Here's how the part is built. I have some questions about the finished solid (model axes, mm). Face numbers are marked on the shaded views. A direction names the side the tool comes from. Coordinates: 2 decimals unless noted, no trailing zeros. Order: outer loops, then holes, each group sorted by start corner. A loop starts at its lowest first (then second) coordinate and runs counter-clockwise, first axis right, second up. Notation, with made-up numbers: (-3, 84) - (25, 84) arc R22 cw to (25, 113) - close; hole circle Ø1 at (3, 61.25). An arc over 180 degrees is marked (long way). Answer in a Markdown table with one row per item. Add a question column.
Item 1: Will these pins go through, and if not, where does the flat tip stop? pin 1 Ø1 at (x, z) = (31.5, -20) entering from +Y; pin 2 Ø2 at (x, z) = (35, 1) entering from +Y; pin 3 Ø1.6 at (x, z) = (14.5, -32.5) entering from +Y.
Item 2: I want a section at A-A (z = 0). Please give me the cut outline in (x, y).
Item 3: I want a section at D-D (z = -30). Please give me the cut outline in (x, y), plus the area to 3 significant figures.
Item 4: I want a section at B-B (y = 5.5). Please give me the cut outline in (x, z) (3 decimals), plus the area to 3 significant figures.
Item 5: If I drill on line 1 along X through (y, z) = (0.7, 0); line 2 along X through (y, z) = (10.16, 10.5); line 3 along Z through (x, y) = (4.5, 15.5), over which ranges is the centre line in solid material (lowest first)? Write a range as from..to.
Item 6: I want a section at C-C (x = 38). Please give me the cut outline in (y, z) (3 decimals), plus the area to 3 significant figures.
Item 7: Thinking about a two-plate mould opening in X: for the marked faces 1, 2 and 3, which applies, +X half, -X half, draft (parallel to the pull), parting line (faces both ways), or undercut?
Item 8: On a 3-axis mill with a long thin cutter (end or side, diameter ignored), from which of +Z, -Z, +X, -X, +Y, -Y can I reach the whole of each face in a straight line? I mean the marked faces 4 and 5. Say none if no direction works.
```python
from build123d import *

# Parameters (mm, degrees)
SKETCH1_W               = 40.64
SKETCH1_H               = 17.526
BOSS_EXTRUDE1_DEPTH     = 37.211
CUT_EXTRUDE1_DEPTH      = 32.385
FILLET1_R               = 3.81
SKETCH3_W               = 3.175
SKETCH3_H               = 6.35
SKETCH3_W_2             = 19.05
CUT_EXTRUDE2_DEPTH      = 58.822390101
CHAMFER1_SIZE           = 10
CUT_EXTRUDE7_DEPTH      = 58.822390101
CUT_EXTRUDE7_DEPTH_BACK = 58.822390101
SKETCH5_R               = 1.5875
BOSS_EXTRUDE2_REACH     = 83.728
SKETCH6_W               = 2.032
SKETCH6_H               = 6.35
BOSS_EXTRUDE3_REACH     = 83.728
SKETCH7_W               = 2.032
SKETCH7_H               = 6.35


with BuildPart() as part:
    # Sketch1 → Boss-Extrude1 (new, symmetric)
    with BuildSketch(Plane.XY):
        with Locations((20.32, 8.763)):
            Rectangle(SKETCH1_W, SKETCH1_H)
    extrude(amount=BOSS_EXTRUDE1_DEPTH, both=True)

    # Sketch2 → Cut-Extrude1 (cut, symmetric)
    with BuildSketch(Plane.XY):
        with BuildLine():
            Line((19.304, 10.16), (19.304, 17.526))
            Line((19.304, 17.526), (15.578005168, 17.526))
            ThreePointArc((15.578005168, 17.526), (2.000497097, 6.032622095), (19.304, 10.16))
        make_face()
        with BuildLine():
            Line((21.336, 10.16), (21.336, 17.526))
            Line((21.336, 17.526), (25.061994832, 17.526))
            ThreePointArc((25.061994832, 17.526), (38.639502903, 6.032622095), (21.336, 10.16))
        make_face()
    extrude(amount=CUT_EXTRUDE1_DEPTH, both=True, mode=Mode.SUBTRACT)

    # Fillet1
    fillet1_edges = [part.edges().sort_by_distance(p)[0] for p in [
        (0, 17.526, 0),
        (40.64, 17.526, 0),
    ]]
    fillet(fillet1_edges, radius=FILLET1_R)

    # Sketch3 → Cut-Extrude2 (cut, through all)
    with BuildSketch(Plane(origin=(40.64, 0, 0), x_dir=(0, 0, -1), z_dir=(1, 0, 0))):
        with Locations((-33.0835, 14.351)):
            Rectangle(SKETCH3_W, SKETCH3_H)
        with Locations((0, 14.351)):
            Rectangle(SKETCH3_W_2, SKETCH3_H)
        with Locations((33.0835, 14.351)):
            Rectangle(SKETCH3_W, SKETCH3_H)
    extrude(amount=-CUT_EXTRUDE2_DEPTH, mode=Mode.SUBTRACT)

    # Chamfer1
    # the kernel refuses this chamfer: 10 mm, written as the material it takes off along each edge
    with BuildSketch(Plane(origin=(21.336, 17.526, -9.525), x_dir=(0, -0.9996219169112968, 0.027495876610586664), z_dir=(-1, 0, 0))) as chamfer1_piece_1_section:
        Polygon((CHAMFER1_SIZE * 0.999621916911, -CHAMFER1_SIZE * 0.0274958766106), (-CHAMFER1_SIZE * 0.0274958766106, -CHAMFER1_SIZE * 0.999621916911), (0, 0), align=None)
    chamfer1_piece_1 = extrude(amount=2.032, mode=Mode.PRIVATE)
    chamfer1_piece_1 = split(chamfer1_piece_1, bisect_by=Plane(origin=(20.32, 11.176, -13.183669109), z_dir=(0, 1, 0)), keep=Keep.TOP, mode=Mode.PRIVATE)
    add(chamfer1_piece_1, mode=Mode.SUBTRACT)
    with BuildSketch(Plane(origin=(21.336, 17.526, 9.525), x_dir=(0, 0.027495876610586324, 0.9996219169112968), z_dir=(-1, 0, 0))) as chamfer1_piece_2_section:
        Polygon((CHAMFER1_SIZE * 0.999621916911, -CHAMFER1_SIZE * 0.0274958766106), (-CHAMFER1_SIZE * 0.0274958766106, -CHAMFER1_SIZE * 0.999621916911), (0, 0), align=None)
    chamfer1_piece_2 = extrude(amount=2.032, mode=Mode.PRIVATE)
    chamfer1_piece_2 = split(chamfer1_piece_2, bisect_by=Plane(origin=(20.32, 11.176, 13.183669109), z_dir=(0, 1, 0)), keep=Keep.TOP, mode=Mode.PRIVATE)
    add(chamfer1_piece_2, mode=Mode.SUBTRACT)

    # Sketch5 → Cut-Extrude7 (cut, two sides: drawn at the far end of the back side and taken through both)
    with BuildSketch(Plane.XZ.offset(-CUT_EXTRUDE7_DEPTH_BACK)):
        with Locations(Location((30.423380261, 0, 0), (0, 0, 270))):
            Circle(SKETCH5_R)
        with Locations(Location((10.216619739, 0, 0), (0, 0, 270))):
            Circle(SKETCH5_R)
    extrude(amount=CUT_EXTRUDE7_DEPTH + CUT_EXTRUDE7_DEPTH_BACK, mode=Mode.SUBTRACT)

    # Sketch6 → Boss-Extrude2 (add, up to next)
    with BuildSketch(Plane(origin=(0, 0, -31.496), x_dir=(-1, 0, 0), z_dir=(0, 0, -1)), mode=Mode.PRIVATE) as boss_extrude2_sk1:
        with Locations((-20.32, 14.351)):
            Rectangle(SKETCH6_W, SKETCH6_H)
    boss_extrude2_tool1 = extrude(boss_extrude2_sk1.sketch, amount=BOSS_EXTRUDE2_REACH, mode=Mode.PRIVATE) - part.part
    add(boss_extrude2_tool1.solids().sort_by_distance((20.32, 14.351, -31.496))[0])

    # Sketch7 → Boss-Extrude3 (add, up to next)
    with BuildSketch(Plane.XY.offset(31.496), mode=Mode.PRIVATE) as boss_extrude3_sk1:
        with Locations((20.32, 14.351)):
            Rectangle(SKETCH7_W, SKETCH7_H)
    boss_extrude3_tool1 = extrude(boss_extrude3_sk1.sketch, amount=BOSS_EXTRUDE3_REACH, mode=Mode.PRIVATE) - part.part
    add(boss_extrude3_tool1.solids().sort_by_distance((20.32, 14.351, 31.496))[0])


solid = part.part
```
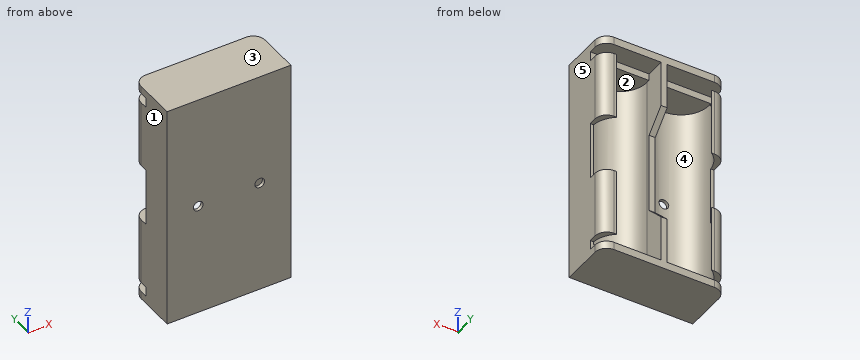
Values follow:
| question | item | result |
|---|---|---|
| 1 | pin 1 | stops at y = 1.14 |
| 1 | pin 2 | stops at y = 2.87 |
| 1 | pin 3 | stops at y = 11.18 |
| 2 | outline | (0, 0) - (8.63, 0) - (8.63, 1.15) arc R9.14 cw to (1.07, 11.18) - (0, 11.18) - close; (11.8, 0) - (28.84, 0) - (28.84, 1.17) arc R9.14 cw to (21.34, 10.16) - (21.34, 11.18) - (19.3, 11.18) - (19.3, 10.16) arc R9.14 cw to (11.8, 1.17) - close; (32.01, 0) - (40.64, 0) - (40.64, 11.18) - (39.57, 11.18) arc R9.14 cw to (32.01, 1.15) - close |
| 3 | outline | (0, 0) - (40.64, 0) - (40.64, 13.72) arc R3.81 ccw to (36.83, 17.53) - (35.9, 17.53) arc R9.14 cw (long way) to (21.34, 10.16) - (21.34, 17.53) - (19.3, 17.53) - (19.3, 10.16) arc R9.14 cw (long way) to (4.74, 17.53) - (3.81, 17.53) arc R3.81 ccw to (0, 13.72) - close |
| 3 | area | 190 mm^2 |
| 4 | outline | (0, -37.211) - (40.64, -37.211) - (40.64, 37.211) - (0, 37.211) - close; hole (2.293, -32.385) - (18.027, -32.385) - (18.027, 32.385) - (2.293, 32.385) - close; hole (22.613, -32.385) - (38.347, -32.385) - (38.347, 32.385) - (22.613, 32.385) - close |
| 4 | area | 986 mm^2 |
| 5 | line 1 | x = 0..8.63, 11.8..28.84, 32.01..40.64 |
| 5 | line 2 | x = 0..1.02, 19.3..21.34, 39.62..40.64 |
| 5 | line 3 | z = -37.21..-34.67, 34.67..37.21 |
| 6 | outline | (0, -37.211) - (17.342, -37.211) - (17.342, -34.671) - (11.176, -34.671) - (11.176, -32.385) - (4.958, -32.385) - (4.958, 32.385) - (11.176, 32.385) - (11.176, 34.671) - (17.342, 34.671) - (17.342, 37.211) - (0, 37.211) - close; (15.362, -31.496) - (17.342, -31.496) - (17.342, -9.525) - (15.362, -9.525) - close; (15.362, 9.525) - (17.342, 9.525) - (17.342, 31.496) - (15.362, 31.496) - close |
| 6 | area | 547 mm^2 |
| 7 | face 1 | -X half |
| 7 | face 2 | undercut |
| 7 | face 3 | draft |
| 8 | face 4 | none |
| 8 | face 5 | +Z, -Z, +X, +Y, -Y |
